Here's how the part is built. I have some questions about the finished solid (model axes, mm). Face numbers are marked on the shaded views. A direction names the side the tool comes from. Give positions to 0.01 mm unless a question says otherwise; leave off trailing zeros. Loops run counter-clockwise (first coordinate to the right, second up) from the corner with the lowest first, then second, coordinate; pieces in that order, holes last. Notation, with made-up numbers: (-38.75, -8) - (16.25, -8) arc R29 ccw to (16.25, 14) - close; hole circle Ø5 at (63.5, 76.25). An arc over 180 degrees is marked (long way). Use one line per item in the form item = value.
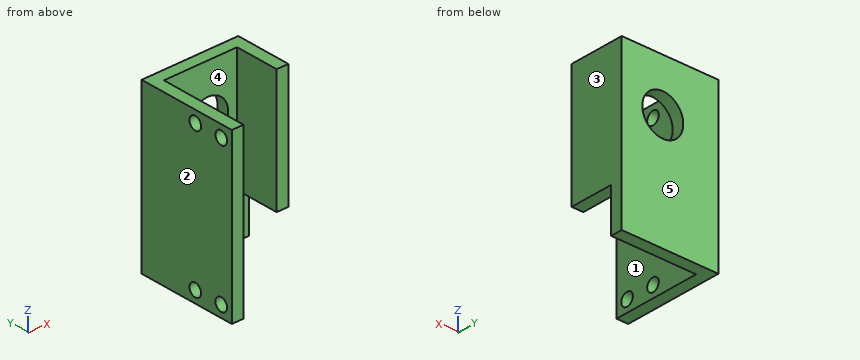
from build123d import *

# Parameters (mm, degrees)
SKETCH1_W           = 57.02
SKETCH1_H           = 34.2
SKETCH1_R           = 2.2
BOSS_EXTRUDE1_DEPTH = 4
SKETCH2_W           = 57.02
SKETCH2_H           = 4
BOSS_EXTRUDE2_DEPTH = 29.05
SKETCH3_W           = 4
SKETCH3_H           = 42.02
BOSS_EXTRUDE3_DEPTH = 15
SKETCH5_R           = 7
CUT_EXTRUDE1_DEPTH  = 4


with BuildPart() as part:
    # Sketch1 → Boss-Extrude1 (new body)
    with BuildSketch(Plane(origin=(0, 0, 0), x_dir=(0, 0, -1), z_dir=(1, 0, 0))):
        Rectangle(SKETCH1_W, SKETCH1_H)
        with Locations((-24.51, -3.25)):
            Circle(SKETCH1_R, mode=Mode.SUBTRACT)
        with Locations((-24.51, -13.1)):
            Circle(SKETCH1_R, mode=Mode.SUBTRACT)
        with Locations((24.51, -3.25)):
            Circle(SKETCH1_R, mode=Mode.SUBTRACT)
        with Locations((24.51, -13.1)):
            Circle(SKETCH1_R, mode=Mode.SUBTRACT)
    extrude(amount=BOSS_EXTRUDE1_DEPTH)

    # Sketch2 → Boss-Extrude2 (add)
    with BuildSketch(Plane(origin=(4, 0, 0), x_dir=(0, 0, -1), z_dir=(1, 0, 0))):
        with Locations((0, 15.1)):
            Rectangle(SKETCH2_W, SKETCH2_H)
    extrude(amount=BOSS_EXTRUDE2_DEPTH)

    # Sketch3 → Boss-Extrude3 (add)
    with BuildSketch(Plane.XZ.offset(-13.1)):
        with Locations((31.05, 7.5)):
            Rectangle(SKETCH3_W, SKETCH3_H)
    extrude(amount=BOSS_EXTRUDE3_DEPTH)

    # Sketch5 → Cut-Extrude1 (cut)
    with BuildSketch(Plane(origin=(0, 17.1, 0), x_dir=(1, 0, 0), z_dir=(0, 1, 0))):
        with Locations((19, -10.79)):
            Circle(SKETCH5_R)
    extrude(amount=-CUT_EXTRUDE1_DEPTH, mode=Mode.SUBTRACT)


solid = part.part
(1) If we section it at A-A (z = 10.79): List the corners of the cut face in (x, y) for me.
Geometry says:
outline = (0, -17.1) - (4, -17.1) - (4, 13.1) - (12, 13.1) - (12, 17.1) - (0, 17.1) - close; (26, 13.1) - (29.05, 13.1) - (29.05, -1.9) - (33.05, -1.9) - (33.05, 17.1) - (26, 17.1) - close
(2) If I drill on probe 1 along Z at (x, y) = (2, -13); probe 2 along X at (y, z) = (3.5, 10); probe 3 along Y at (x, z) = (1, -24), over which ranges is the centre line in solid material (lowest first)?
Geometry says:
probe_1 = -28.51 to -26.71, -22.31 to 22.31, 26.71 to 28.51
probe_2 = 0 to 4, 29.05 to 33.05
probe_3 = -17.1 to -15.24, -10.96 to -5.39, -1.11 to 17.1
(3) Thinking about a two-plate mould opening in X: for the marked faces 3, 4 and 5, which applies, pulls with the +X half, pulls with the -X half, needs draft (parallel to the pull), parting line crosses it, or undercut?
Geometry says:
face_3 = pulls with the +X half
face_4 = undercut
face_5 = needs draft
(4) If we section it at D-D (z = -24.51): List the corners of the cut face in (x, y) for me.
Geometry says:
outline = (0, -17.1) - (4, -17.1) - (4, -15.3) - (0, -15.3) - close; (0, -10.9) - (4, -10.9) - (4, -5.45) - (0, -5.45) - close; (0, -1.05) - (4, -1.05) - (4, 13.1) - (33.05, 13.1) - (33.05, 17.1) - (0, 17.1) - close
(5) For the marked faces 1 and 2, which set-ups out of +Z, -Z, +X, -X, +Y, -Y let a thin tool reach every point of the face, with its end or its side?
Geometry says:
face_1 = +Z, -Z, -Y
face_2 = +Z, -Z, -X, +Y, -Y
(6) If we section it at C-C (y = 3.5): List the corners of the cut face in (x, z) for me.
Geometry says:
outline = (0, -28.51) - (4, -28.51) - (4, 28.51) - (0, 28.51) - close; (29.05, -13.51) - (33.05, -13.51) - (33.05, 28.51) - (29.05, 28.51) - close
(7) For P1, Ø2, axis at x = 30, z = 14.5, coming from the -Y side; P2, Ø6, axis at x = 18, z = -7, coming from the -Y side; P3, Ø4, axis at y = -6.5, z = 22, coming from the +X side, each with a flat end and sliding along its axis, tell me the tip position at first contact or that it passes through.
Geometry says:
P1 = -1.9
P2 = 13.1
P3 = 4
(8) If we section it at B-B (x = 19): List the corners of the cut face in (y, z) for me, plus the area to 3 significant figures.
Geometry says:
outline = (13.1, -28.51) - (17.1, -28.51) - (17.1, 3.79) - (13.1, 3.79) - close; (13.1, 17.79) - (17.1, 17.79) - (17.1, 28.51) - (13.1, 28.51) - close
area = 172 mm²
